from build123d import *

# Parameters (mm, degrees)
F0_W = 7
F0_H = 6


with BuildPart() as f2:
    # F2: sweep along a path in F1
    with BuildLine(Plane.XY) as f2_path:
        Line((0, 0), (0, -60.457104))
        ThreePointArc((0, -60.457104), (0.626434, -62.606303), (2.309527, -64.082335))
        Line((2.309527, -64.082335), (15, -70))
    # F0 (on Front) → F2 (sweep)
    with BuildSketch(Plane.XZ):
        Rectangle(F0_W, F0_H)
    sweep(path=f2_path.line)


solid = f2.part
Geometry check sheet. Reference: the model listing, model coordinates, mm. A direction names the side the tool comes from. Give positions to 0.01 mm unless a question says otherwise; leave off trailing zeros. Write each loop counter-clockwise with the first axis right and the second up, starting at its lowest first coordinate (ties: lowest second). Pieces come first, ordered by that corner, then holes.
1) Thickness scan on line 1 (X direction, y = -5, z = 1.85); line 2 (Y direction, x = 5, z = 0.15); line 3 (Y direction, x = 12.25, z = -2.5). Record the ranges inside material, lowest first.
Values follow:
line 1: x = -3.5 to 3.5
line 2: y = -69.2 to -61.48
line 3: y = -72.58 to -64.86
2) Set-up check for faces 1 (the face through (3.5, -31, 0)), 2 (the face through (3, -39, -3)): record each of +Z, -Z, +X, -X, +Y, -Y from which the full face is reachable in a straight line by a thin tool's end or side.
Values follow:
face 1: +Z, -Z, +X, +Y
face 2: -Z, +X, -X, +Y, -Y
3) Cross-section at C-C (y = -18). Record the boundary of the cut face in (x, z), plus the area to 3 significant figures.
Values follow:
outline: (-3.5, -3) - (3.5, -3) - (3.5, 3) - (-3.5, 3) - close
area: 42.0 mm2
4) Cross-section at A-A (z = -1.65). Record the boundary of the cut face in (x, y), plus the area to 3 significant figures.
Values follow:
outline: (-3.5, -60.46) arc R7.5 ccw to (0.83, -67.25) - (13.52, -73.17) - (16.48, -66.83) - (3.79, -60.91) arc R0.5 cw to (3.5, -60.46) - (3.5, 0) - (-3.5, 0) - close
area: 553 mm2
5) Cross-section at B-B (x = 2.25). Record the boundary of the cut face in (y, z).
Values follow:
outline: (-67.92, -3) - (0, -3) - (0, 3) - (-67.92, 3) - close
6) Go/stop test with a flat-tipped pin: pin 1 Ø2 at (y, z) = (-32.5, 1) entering from +X. Record where the tip stops, or that it passes through.
Values follow:
pin 1: stops at x = 3.5
